```python
from build123d import *

# Parameters (mm, degrees)
F1_DEPTH = 25.4
F2_DEPTH = 42.9268069565
F3_DEPTH = 118.9797818661


# Not quite as in the source:
# - the program builds the solid bodies; features that only make, move or delete a surface that nothing else refers to are left out


with BuildPart() as f1:
    # F0 (on Front) → F1 (new body)
    with BuildSketch(Plane.XZ):
        Polygon((39.7322513163, -37.4155193567), (36.51605919, 29.1617289186), (-39.3116846681, 29.1617289186), (-42.4041748047, -32.5892791152), align=None)
    extrude(amount=F1_DEPTH)

    # F2 (add): a face of the model
    f2_faces = [f1.faces().sort_by_distance(p)[0] for p in [
        (-0.8911665314, -25.4, -3.3616464638),
    ]]
    extrude(f2_faces, amount=F2_DEPTH)

    # F3 (add): faces of the model
    f3_faces = [f1.faces().sort_by_distance(p)[0] for p in [
        (-1.397812739, -34.1634034783, 29.1617289186),
        (38.1241552532, -34.1634034783, -4.1268952191),
        (-1.3359617442, -34.1634034783, -35.002399236),
    ]]
    extrude(f3_faces, amount=-F3_DEPTH, dir=(0, 0, 1))


solid = f1.part
```
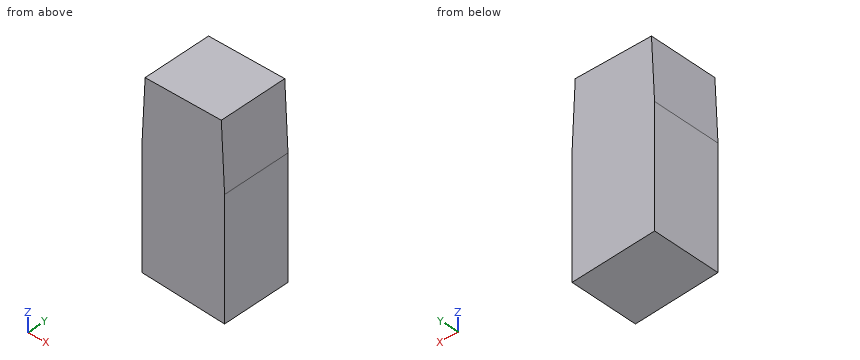
Here's how the part is built. I have some questions about the finished solid (model axes, mm). Coordinates: 2 decimals unless noted, no trailing zeros. Write each loop counter-clockwise with the first axis right and the second up, starting at its lowest first coordinate (ties: lowest second). Pieces come first, ordered by that corner, then holes. Notation, with made-up numbers: M 15.25,-38.75 L 63.25,-38.75 A11 cw 63.25,-18.75 Z; hole C 77.25,-18.5 d11. An arc over 180 degrees is marked long. Answer as CSV lines item,"result". Start each with the question number.
Q1. Suppose I cut it at B-B, the plane x = -27. List the corners of the cut face in (y, z) for me.
Q2. I need wall thicknesses on probe 1 along X at (y, z) = (-43, 18); probe 2 along X at (y, z) = (-56, 11.5); probe 3 along Z at (x, y) = (6.5, -58). Which ranges of each line are inside material? Lowest first, please. Write a range as [from, to].
Q3. Will these pins go through, and if not, where does the flat tip stop? pin 1 Ø3 at (x, y) = (-18, -51.5) entering from -Z; pin 2 Ø12 at (y, z) = (-15.5, -25.5) entering from -X; pin 3 Ø12 at (y, z) = (-31.5, 10) entering from +X.
Q4. Suppose I cut it at C-C, the plane z = 11. List the corners of the cut face in (x, y) for me.
Q5. Suppose I cut it at A-A, the plane y = -29. List the corners of the cut face in (x, z) for me.
Entries:
1,outline,"M -68.33,-152.47 L 0,-152.47 L 0,29.16 L -68.33,29.16 Z"
2,probe 1,"x = [-39.87, 37.06]"
2,probe 2,"x = [-40.2, 37.37]"
2,probe 3,"z = [-154.44, 29.16]"
3,pin 1,"stops at z = -153.09"
3,pin 2,"stops at x = -42.35"
3,pin 3,"stops at x = 37.73"
4,outline,"M -40.22,-68.33 L 37.39,-68.33 L 37.39,0 L -40.22,0 Z"
5,outline,"M -42.4,-151.57 L 39.73,-156.4 L 39.73,-37.42 L 36.52,29.16 L -39.31,29.16 L -42.4,-32.59 Z"
